from build123d import *

# Parameters (mm, degrees)
BOSS_EXTRUDE1_DEPTH = 38.1
SKETCH2_R           = 3.3655
CUT_EXTRUDE1_DEPTH  = 12.557


with BuildPart() as part:
    # Sketch1 → Boss-Extrude1 (new body)
    with BuildSketch(Plane(origin=(0, 0, 0), x_dir=(0, 0, -1), z_dir=(1, 0, 0))):
        Polygon((0, 0), (0, -38.1), (-9.525, -38.1), (-9.525, -76.2), (-7.493, -76.2), (-7.493, -40.132), (2.032, -40.132), (2.032, 0), align=None)
    extrude(amount=BOSS_EXTRUDE1_DEPTH)

    # Sketch2 → Cut-Extrude1 (cut, through all)
    with BuildSketch(Plane.XY.offset(9.525)):
        with Locations((9.525, -66.675)):
            Circle(SKETCH2_R)
        with Locations((28.575, -47.625)):
            Circle(SKETCH2_R)
    extrude(amount=-CUT_EXTRUDE1_DEPTH, mode=Mode.SUBTRACT)


solid = part.part
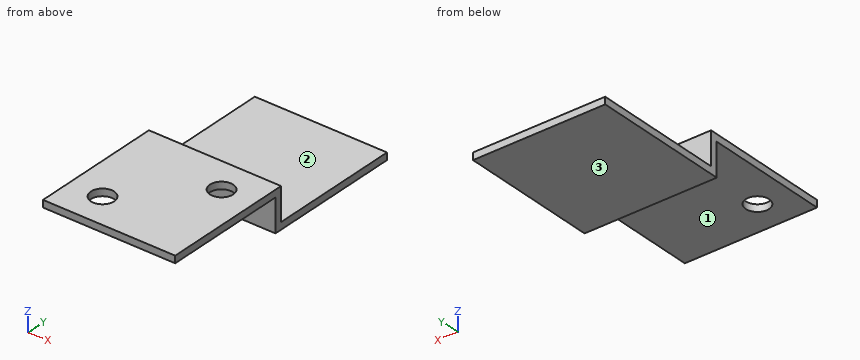
Here's how the part is built. I have some questions about the finished solid (model axes, mm). Face numbers are marked on the shaded views. A direction names the side the tool comes from. Give positions to 0.01 mm unless a question says otherwise; leave off trailing zeros. Write each loop counter-clockwise with the first axis right and the second up, starting at its lowest first coordinate (ties: lowest second). Pieces come first, ordered by that corner, then holes. Notation, with made-up numbers: (-32, 5) -> (18, 5) arc R22 cw to (18, 17) -> close; hole circle Ø7 at (13, 18.25). An arc over 180 degrees is marked (long way). Use one line per item in the form item = value. Start each with the question number.
1. Will these pins go through, and if not, where does the flat tip stop? pin 1 Ø5 at (x, z) = (13, 3) entering from +Y; pin 2 Ø3 at (x, z) = (19, 5) entering from -Y; pin 3 Ø10 at (x, y) = (12, -54.5) entering from -Z.
2. Imagine slicing it at C-C on y = -58.5. List the corners of the cut face in (x, z) for me (3 decimals).
3. If I drill on L1, parallel to Z at x = 34.5, y = -44 (3 decimals); L2, parallel to Y at x = 20, z = 5.75; L3, parallel to Z at x = 15.5, y = -26.5, over which ranges is the centre line in solid material (lowest first)?
4. Imagine slicing it at D-D on z = 8.5. List the corners of the cut face in (x, y) for me (1 decimal), plus the area to 3 significant figures.
5. Imagine slicing it at A-A on x = 26. List the corners of the cut face in (y, z) for me (3 decimals).
6. Imagine slicing it at B-B on x = 22. List the corners of the cut face in (y, z) for me (3 decimals).
7. On a 3-axis mill with a long thin cutter (end or side, diameter ignored), from which of +Z, -Z, +X, -X, +Y, -Y can I reach the whole of each face in a straight line? I mean the marked faces 1, 2 and 3. Say none if no direction works.
Entries:
q1.pin_1 = -38.1
q1.pin_2 = -40.13
q1.pin_3 = 7.49
q2.outline = (0, 7.493) -> (38.1, 7.493) -> (38.1, 9.525) -> (0, 9.525) -> close
q3.L1 = 7.493 to 9.525
q3.L2 = -40.13 to -38.1
q3.L3 = -2.03 to 0
q4.outline = (0, -76.2) -> (38.1, -76.2) -> (38.1, -38.1) -> (0, -38.1) -> close; hole circle Ø6.7 at (9.5, -66.7); hole circle Ø6.7 at (28.6, -47.6)
q4.area = 1,380 mm²
q5.outline = (-76.2, 7.493) -> (-49.792, 7.493) -> (-49.792, 9.525) -> (-76.2, 9.525) -> close; (-45.458, 7.493) -> (-40.132, 7.493) -> (-40.132, -2.032) -> (0, -2.032) -> (0, 0) -> (-38.1, 0) -> (-38.1, 9.525) -> (-45.458, 9.525) -> close
q6.outline = (-76.2, 7.493) -> (-40.132, 7.493) -> (-40.132, -2.032) -> (0, -2.032) -> (0, 0) -> (-38.1, 0) -> (-38.1, 9.525) -> (-76.2, 9.525) -> close
q7.face_1 = -Z, +X, -X, -Y
q7.face_2 = +Z, +X, -X, +Y
q7.face_3 = -Z, +X, -X, +Y, -Y
